Build history of the part. All positions in model axes, mm. Face numbers are marked on the shaded views. A direction names the side the tool comes from. Coordinates: 2 decimals unless noted, no trailing zeros. Write each loop counter-clockwise with the first axis right and the second up, starting at its lowest first coordinate (ties: lowest second). Pieces come first, ordered by that corner, then holes.
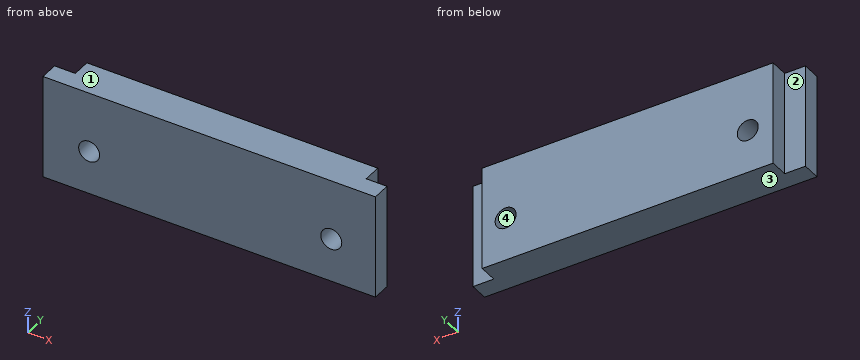
Autodesk Inventor part; units mm, degrees
ref_plane "YZ Plane" through (0, 0, 0) normal (1, 0, 0) x (0, 1, 0)
ref_plane "XZ Plane" through (0, 0, 0) normal (0, 1, 0) x (-1, 0, 0)
ref_plane "XY Plane" through (0, 0, 0) normal (0, 0, 1) x (1, 0, 0)
sketch "Sketch1" plane through (0, 0, 0) normal (0, 1, 0) x (-1, 0, 0)
  line L0 (0, 0) -> (-50.8, 0)
  line L1 (-50.8, 0) -> (-50.8, 15.875)
  line L2 (-50.8, 15.875) -> (0, 15.875)
  line L3 (0, 15.875) -> (0, 0)
  dimension "d0" = 50.8
  dimension "d1" = 15.875
extrude "Extrusion1" add sketch "Sketch1" along normal blind 5.6134
sketch "Sketch7" plane through (0, 5.6134, 0) normal (0, 1, 0) x (1, 0, 0)
  circle A0 centre (7.052, -6.6524) radius 1.6
  circle A1 centre (44.052, -6.6524) radius 1.6
  line L0 (0, 0) -> (0, -15.875)
  line L1 (50.8, 0) -> (0, 0)
  dimension "d22" = 3.2
  dimension "d23" = 3.2
  dimension "d24" = 37
  dimension "d42" = 7.052
  dimension "d43" = 6.6524
  dimension "d44" = 6.6524
extrude "Extrusion6" cut sketch "Sketch7" against normal blind 25.4
sketch "Sketch8" plane through (0, 5.6134, 0) normal (0, 1, 0) x (1, 0, 0)
  line L0 (50.8, 0) -> (0, 0)
  line L1 (0, 0) -> (0, -15.875)
  line L2 (50.8, -15.875) -> (50.8, 0)
  line L3 (0, -15.875) -> (3.175, -15.875)
  line L4 (3.175, -15.875) -> (3.175, 0)
  line L5 (3.175, 0) -> (0, 0)
  line L6 (0, 0) -> (0, -15.875)
  line L7 (50.8, -15.875) -> (47.625, -15.875)
  line L8 (47.625, -15.875) -> (47.625, 0)
  line L9 (47.625, 0) -> (50.8, 0)
  line L10 (50.8, 0) -> (50.8, -15.875)
  dimension "d34" = 3.175
  dimension "d35" = 3.175
extrude "Extrusion7" cut sketch "Sketch8" against normal blind 2.8067
equation "\"d23\" = d22"
properties part number "Lidar Sensor Case Piece 3"
1. Mould opens along X. For the marked faces 3 and 4 say: +X half, -X half, draft (parallel to the pull), parting line (faces both ways), or undercut.
Computed values:
face 3: draft
face 4: undercut
2. Saw through at A-A on z = 1.5. List the corners of the cut face in (x, y) (3 decimals).
Computed values:
outline: (0, 0) - (50.8, 0) - (50.8, 2.807) - (47.625, 2.807) - (47.625, 5.613) - (3.175, 5.613) - (3.175, 2.807) - (0, 2.807) - close
3. 3-axis set-ups, long thin cutter, end or side, ignore diameter. For the marked faces 1 and 2: which of +Z, -Z, +X, -X, +Y, -Y reach the whole face in a straight line?
Computed values:
face 1: +Z, +X, -X, +Y, -Y
face 2: +Z, -Z, -X, +Y
4. Saw through at B-B on x = 8. List the corners of the cut face in (y, z) (3 decimals), plus the area to 3 significant figures.
Computed values:
outline: (0, 0) - (5.613, 0) - (5.613, 5.363) - (0, 5.363) - close; (0, 7.941) - (5.613, 7.941) - (5.613, 15.875) - (0, 15.875) - close
area: 74.6 mm2
5. Saw through at C-C on z = 5.5. List the corners of the cut face in (x, y) (3 decimals).
Computed values:
outline: (0, 0) - (5.942, 0) - (5.942, 5.613) - (3.175, 5.613) - (3.175, 2.807) - (0, 2.807) - close; (8.162, 0) - (42.942, 0) - (42.942, 5.613) - (8.162, 5.613) - close; (45.162, 0) - (50.8, 0) - (50.8, 2.807) - (47.625, 2.807) - (47.625, 5.613) - (45.162, 5.613) - close
6. Probe line 1 along X through (y, z) = (2.4, 6.5); line 2 along Z through (x, y) = (44, 0.75) (3 decimals); line 3 along X through (y, z) = (3.8, 5.75) (3 decimals). List the from-to ranges inside material, lowest first.
Computed values:
line 1: x = 0 to 5.46, 8.64 to 42.46, 45.64 to 50.8
line 2: z = 0 to 5.053, 8.252 to 15.875
line 3: x = 3.175 to 5.731, 8.373 to 42.731, 45.373 to 47.625
7. Flat gauge pins, fed straight in: pin 1 (1 mm diameter, centred on x = 2, z = 9, fed in from +Y); pin 2 (3 mm diameter, centred on y = 2, z = 9.5, fed in from -X); pin 3 (1.4 mm diameter, centred on y = 4.5, z = 4.5, fed in from -X) (3 decimals). Where does each tip first touch, or does it go through?
Computed values:
pin 1: stops at y = 2.81
pin 2: stops at x = 0
pin 3: stops at x = 3.175
8. Saw through at D-D on y = 0.5. List the corners of the cut face in (x, z) (3 decimals).
Computed values:
outline: (0, 0) - (50.8, 0) - (50.8, 15.875) - (0, 15.875) - close; hole circle Ø3.2 at (7.052, 6.652); hole circle Ø3.2 at (44.052, 6.652)
